Input: part model. Units: mm. Frame: model coordinates. A direction names the side the tool comes from. Coordinates: 2 decimals unless noted, no trailing zeros. Loops run counter-clockwise (first coordinate to the right, second up) from the corner with the lowest first, then second, coordinate; pieces in that order, holes last.
(1) Mould query, pull axis Y, two halves, no side actions, for faces 5 (the face through (1, 66, 2)), 6 (the face through (22, 131, 3)), 7 (the face through (22, 24, 5)). Classes: released by +Y, released by -Y, zero draft, split by the parting line, or undercut.
(2) Line query: L1, parallel to Y at x = 27.5, z = 2.75; L2, parallel to X at y = 108.5, z = -2; L3, parallel to X at y = 89, z = 4.25. Output: solid intervals per line, ascending.
(3) Set-up query: faces 1 (the face through (22, 119, 5)), 2 (the face through (22, 118, -2)), 3 (the face through (30, 72, 0)), 4 (the face through (44, 66, 2)). Return all of +Z, -Z, +X, -X, +Y, -Y with unobstructed straight access to the full face (end or side cutting, diameter ignored); none if empty.
(4) Section A-A, the plane x = 33. Return loops of the section in (y, z), then the cut area to 3 significant figures.
(5) Contact query for flat-ended pins moving along their axis: P1, Ø3, axis at y = 51, z = 5, coming from the -X side; P2, Ø4.5, axis at x = 16, y = 70, coming from the +Z side; P3, Ø0.6, axis at y = 23.5, z = 3.5, coming from the +X side. Output: stop coordinate, or through.
(6) Section B-B, the plane y = 36.5. Return loops of the section in (x, z).
```python
from build123d import *

# Parameters (mm, degrees)
F0_W      = 45
F0_H      = 131
F1_DEPTH  = 2
F2_W      = 40.5
F2_H      = 131
F3_DEPTH  = 5
F5_W      = 35
F5_H      = 100
F6_DEPTH  = 4
F7_W      = 5
F7_H      = 100
F8_DEPTH  = 2
F4_W      = 15
F4_H      = 90
F9_DEPTH  = 7.001
F10_W     = 5
F10_H     = 5
F13_DEPTH = 2
F12_W     = 5
F12_H     = 5
F14_DEPTH = 4
F11_W     = 10
F11_H     = 100
F15_DEPTH = 4
F16_R     = 1.5
F17_DEPTH = 131.001


with BuildPart() as f1:
    # F0 (on Top) → F1 (new body)
    with BuildSketch(Plane.XY):
        with Locations((22.5, 65.5)):
            Rectangle(F0_W, F0_H)
    extrude(amount=F1_DEPTH)

    # F2 (on face) → F3 (join)
    with BuildSketch(Plane.XY.offset(2)):
        with Locations((22.5, 65.5)):
            Rectangle(F2_W, F2_H)
    extrude(amount=F3_DEPTH)

    # F5 (on face) → F6 (cut)
    with BuildSketch(Plane.XY.offset(7)):
        with Locations((22.5, 71)):
            Rectangle(F5_W, F5_H)
    extrude(amount=-F6_DEPTH, mode=Mode.SUBTRACT)

    # F7 (on face) → F8 (join)
    with BuildSketch(Plane.XY.offset(3)):
        with Locations((22.5, 71)):
            Rectangle(F7_W, F7_H)
    extrude(amount=F8_DEPTH)

    # F4 (on face) → F9 (cut, through all)
    with BuildSketch(Plane.XY.offset(7)):
        with Locations((22.5, 71)):
            Rectangle(F4_W, F4_H)
    extrude(amount=-F9_DEPTH, mode=Mode.SUBTRACT)

    # F10 (on face) → F13 (join)
    with BuildSketch(Plane(origin=(0, 0, 0), x_dir=(1, 0, 0), z_dir=(0, 0, -1))):
        with Locations((22.5, -118.5)):
            Rectangle(F10_W, F10_H)
        with Locations((22.5, -23.5)):
            Rectangle(F10_W, F10_H)
    extrude(amount=F13_DEPTH)

    # F12 (on face) → F14 (join)
    with BuildSketch(Plane(origin=(0, 0, 0), x_dir=(1, 0, 0), z_dir=(0, 0, -1))):
        with Locations((17.5, -23.5)):
            Rectangle(F12_W, F12_H)
        with Locations((27.5, -23.5)):
            Rectangle(F12_W, F12_H)
        with Locations((27.5, -118.5)):
            Rectangle(F12_W, F12_H)
        with Locations((17.5, -118.5)):
            Rectangle(F12_W, F12_H)
    extrude(amount=F14_DEPTH)

    # F11 (on face) → F15 (join)
    with BuildSketch(Plane(origin=(0, 0, 0), x_dir=(1, 0, 0), z_dir=(0, 0, -1))):
        with Locations((10, -71)):
            Rectangle(F11_W, F11_H)
        with Locations((35, -71)):
            Rectangle(F11_W, F11_H)
    extrude(amount=F15_DEPTH)

    # F16 (on face) → F17 (cut, through all)
    with BuildSketch(Plane.XZ):
        with Locations((2.25, 4.5)):
            Circle(F16_R)
        with Locations((42.75, 4.5)):
            Circle(F16_R)
    extrude(amount=-F17_DEPTH, mode=Mode.SUBTRACT)


solid = f1.part
```
Report:
1. face 5: zero draft
1. face 6: released by +Y
1. face 7: undercut
2. L1: y = 0 to 26, 116 to 131
2. L2: x = 5 to 15, 30 to 40
2. L3: x = 3.73 to 5, 40 to 41.27
3. face 1: +Z
3. face 2: -Z, +Y, -Y
3. face 3: +Z, -Z
3. face 4: +Z, +X, +Y, -Y
4. outline: (0, 0) - (21, 0) - (21, -4) - (121, -4) - (121, 0) - (131, 0) - (131, 7) - (121, 7) - (121, 3) - (21, 3) - (21, 7) - (0, 7) - close
4. area: 917 mm2
5. P1: stops at x = 2.25
5. P2: stops at z = 3
5. P3: stops at x = 42
6. outline: (0, 0) - (5, 0) - (5, -4) - (15, -4) - (15, 3) - (5, 3) - (5, 7) - (2.25, 7) - (2.25, 6) arc R1.5 cw to (2.25, 3) - (2.25, 2) - (0, 2) - close; (30, -4) - (40, -4) - (40, 0) - (45, 0) - (45, 2) - (42.75, 2) - (42.75, 3) arc R1.5 cw to (42.75, 6) - (42.75, 7) - (40, 7) - (40, 3) - (30, 3) - close
